Build history of the part. All positions in model axes, mm. Face numbers are marked on the shaded views. A direction names the side the tool comes from. Round coordinates to 2 decimals unless told otherwise and drop trailing zeros. Write each loop counter-clockwise with the first axis right and the second up, starting at its lowest first coordinate (ties: lowest second). Pieces come first, ordered by that corner, then holes. Notation, with made-up numbers: M 10,85 L 28,85 A16 cw 28,97 Z; hole C 32,41.5 d1. An arc over 180 degrees is marked long. Write item = value, one per line.
from build123d import *

# Parameters (mm, degrees)
SKETCH1_W                                           = 57
SKETCH1_H                                           = 30
BOSS_EXTRUDE1_DEPTH                                 = 4
SKETCH3_R                                           = 4
BOSS_EXTRUDE2_DEPTH                                 = 11.2
SKETCH4_R                                           = 6
BOSS_EXTRUDE3_DEPTH                                 = 1
CBORE_FOR_2_BINDING_HEAD_MACHINE_SCREW1_D           = 2.4384
CBORE_FOR_2_BINDING_HEAD_MACHINE_SCREW1_CBORE_D     = 5.55752
CBORE_FOR_2_BINDING_HEAD_MACHINE_SCREW1_CBORE_DEPTH = 2.000000064
FILLET1_R                                           = 5
FILLET2_R                                           = 2
FILLET3_R                                           = 1


with BuildPart() as part:
    # Sketch1 → Boss-Extrude1 (new body)
    with BuildSketch(Plane(origin=(0, 0, 0), x_dir=(1, 0, 0), z_dir=(0, 1, 0))):
        Rectangle(SKETCH1_W, SKETCH1_H)
    extrude(amount=BOSS_EXTRUDE1_DEPTH)

    # Sketch3 → Boss-Extrude2 (add)
    with BuildSketch(Plane(origin=(0, 4, 0), x_dir=(1, 0, 0), z_dir=(0, 1, 0))):
        with Locations(Location((10.18, 2.35, 0), (0, 0, 90))):
            Circle(SKETCH3_R)
    extrude(amount=BOSS_EXTRUDE2_DEPTH)

    # Sketch4 → Boss-Extrude3 (add)
    with BuildSketch(Plane(origin=(0, 4, 0), x_dir=(1, 0, 0), z_dir=(0, 1, 0))):
        with Locations(Location((10.18, 2.35, 0), (0, 0, 90))):
            Circle(SKETCH4_R)
    extrude(amount=BOSS_EXTRUDE3_DEPTH)

    # CBORE for #2 Binding Head Machine Screw1 (through all)
    with Locations(Plane(origin=(0, 4, 0), x_dir=(1, 0, 0), z_dir=(0, 1, 0))):
        with Locations((-23.5, 9.5), (-23.5, -7.5), (23.5, -7.5), (23.5, 9.5)):
            CounterBoreHole(CBORE_FOR_2_BINDING_HEAD_MACHINE_SCREW1_D / 2, CBORE_FOR_2_BINDING_HEAD_MACHINE_SCREW1_CBORE_D / 2, CBORE_FOR_2_BINDING_HEAD_MACHINE_SCREW1_CBORE_DEPTH)

    # Fillet1
    fillet1_edges = [part.edges().sort_by_distance(p)[0] for p in [
        (-28.5, 2, -15),
        (28.5, 2, -15),
        (28.5, 2, 15),
        (-28.5, 2, 15),
    ]]
    fillet(fillet1_edges, radius=FILLET1_R)

    # Fillet2
    fillet2_edges = [part.edges().sort_by_distance(p)[0] for p in [
        (0, 4, 15),
        (-28.5, 4, 0),
        (28.5, 4, 0),
        (0, 4, -15),
        (27.035533906, 4, 13.535533906),
        (27.035533906, 4, -13.535533906),
        (-27.035533906, 4, -13.535533906),
        (-27.035533906, 4, 13.535533906),
    ]]
    fillet(fillet2_edges, radius=FILLET2_R)

    # Fillet3
    fillet3_edges = [part.edges().sort_by_distance(p)[0] for p in [
        (10.18, 15.2, 1.65),
    ]]
    fillet(fillet3_edges, radius=FILLET3_R)


solid = part.part
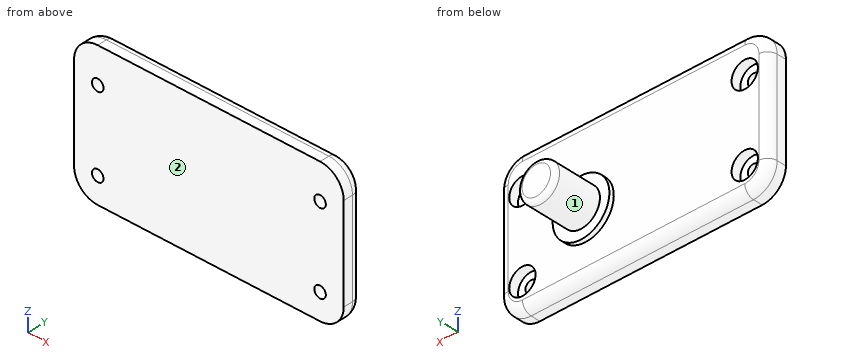
1. Band-saw the part on C-C (y = 12.25). List the corners of the cut face in (x, z), plus the area to 3 significant figures.
Responses:
outline = C 10.18,-2.35 d8
area = 50.3 mm²
2. Tool access for the marked faces 1 and 2: list every direction of +Z, -Z, +X, -X, +Y, -Y with a clear straight run to the whole face (end or side of a thin tool).
Responses:
face_1 = +Y
face_2 = +Z, -Z, +X, -X, -Y
3. Band-saw the part on B-B (x = -2). List the corners of the cut face in (y, z), plus the area to 3 significant figures.
Responses:
outline = M 0,-15 L 2,-15 A2 ccw 4,-13 L 4,13 A2 ccw 2,15 L 0,15 Z
area = 118 mm²
4. Band-saw the part on D-D (x = 10.18). List the corners of the cut face in (y, z), plus the area to 3 significant figures.
Responses:
outline = M 0,-15 L 2,-15 A2 ccw 4,-13 L 4,-8.35 L 5,-8.35 L 5,-6.35 L 14.2,-6.35 A1 ccw 15.2,-5.35 L 15.2,0.65 A1 ccw 14.2,1.65 L 5,1.65 L 5,3.65 L 4,3.65 L 4,13 A2 ccw 2,15 L 0,15 Z
area = 211 mm²
5. Flat gauge pins, fed straight in: pin 1 (9 mm diameter, centred on x = -23.5, z = 7.5, fed in from +Y); pin 2 (3 mm diameter, centred on x = 22.5, z = -9, fed in from +Y); pin 3 (1 mm diameter, centred on x = -2.5, y = 3, fed in from +Z); pin 4 (6 mm diameter, centred on y = 12, z = -12, fed in from +X). Where does each tip first touch, or does it go through?
Responses:
pin_1 = 4
pin_2 = 2
pin_3 = 14.94
pin_4 = through
6. Probe probe 1 along Z at (x, y) = (-23.5, 0.6); probe 2 along X at (y, z) = (0.6, -9.5); probe 3 along Z at (x, y) = (23.5, 2.65). List the from-to ranges inside material, lowest first.
Responses:
probe_1 = -15 to -10.72, -8.28 to 6.28, 8.72 to 15
probe_2 = -28.5 to -24.72, -22.28 to 22.28, 24.72 to 28.5
probe_3 = -14.89 to -12.28, -6.72 to 4.72, 10.28 to 14.89
7. Band-saw the part on A-A (z = -2.35). List the corners of the cut face in (x, y), plus the area to 3 significant figures.
Responses:
outline = M -28.5,0 L 28.5,0 L 28.5,2 A2 ccw 26.5,4 L 16.18,4 L 16.18,5 L 14.18,5 L 14.18,14.2 A1 ccw 13.18,15.2 L 7.18,15.2 A1 ccw 6.18,14.2 L 6.18,5 L 4.18,5 L 4.18,4 L -26.5,4 A2 ccw -28.5,2 Z
area = 319 mm²
